from build123d import *

# Parameters (mm, degrees)
F1_DEPTH = 180
F2_R     = 6.5
F3_DEPTH = 25


with BuildPart() as f1:
    # F0 (on Right) → F1 (new body, symmetric)
    with BuildSketch(Plane.YZ):
        Polygon((-50, 0), (0, 0), (0, 50), (-5, 50), (-5, 5), (-45, 5), (-45, 50), (-50, 50), align=None)
    extrude(amount=F1_DEPTH, both=True)

    # F2 (on face) → F3 (cut)
    with BuildSketch(Plane(origin=(0, 0, 0), x_dir=(1, 0, 0), z_dir=(0, 0, -1))):
        with Locations((-60, 25)):
            Circle(F2_R)
        with Locations((60, 25)):
            Circle(F2_R)
    extrude(amount=-F3_DEPTH, mode=Mode.SUBTRACT)


solid = f1.part
Model file for the job. Use its own axes, mm. A direction names the side the tool comes from. Round coordinates to 2 decimals unless told otherwise and drop trailing zeros. Order: outer loops, then holes, each group sorted by start corner. A loop starts at its lowest first (then second) coordinate and runs counter-clockwise, first axis right, second up.
(1) Pin check, flat tip, straight feed: pin 1 (8 mm diameter, centred on x = 113, y = -19, fed in from +Z). Stop position of the tip, or through.
(2) Drill centre lines: line 1 (X direction, y = -25, z = 2.1); line 2 (Y direction, x = 60, z = 2.6); line 3 (Y direction, x = -85, z = 20). Where is each one in solid material? Low to high.
(3) 3-axis set-ups, long thin cutter, end or side, ignore diameter. For faces 1 (the face through (-180, -25.1, 4.7)), 2 (the face through (3, -45, 27)): which of +Z, -Z, +X, -X, +Y, -Y reach the whole face in a straight line?
(4) Band-saw the part on C-C (z = 15). List the corners of the cut face in (x, y).
(5) Pull direction Y, two halves, no side cores. Call faces 3 (the face through (3, -50, 25)), 4 (the face through (3, -25, 0)), 5 (the face through (-53.8, -26.95, 2.46)): released by +Y, released by -Y, zero draft, split by the parting line, or undercut.
(6) Band-saw the part on B-B (x = -60). List the corners of the cut face in (y, z), then the cut area to 3 significant figures.
(7) Band-saw the part on A-A (y = -25). List the corners of the cut face in (x, z).
Verdict:
1. pin 1: stops at z = 5
2. line 1: x = -180 to -66.5, -53.5 to 53.5, 66.5 to 180
2. line 2: y = -50 to -31.5, -18.5 to 0
2. line 3: y = -50 to -45, -5 to 0
3. face 1: +Z, -Z, -X, +Y, -Y
3. face 2: +Z, +X, -X
4. outline: (-180, -50) - (180, -50) - (180, -45) - (-180, -45) - close; (-180, -5) - (180, -5) - (180, 0) - (-180, 0) - close
5. face 3: released by -Y
5. face 4: zero draft
5. face 5: undercut
6. outline: (-50, 0) - (-31.5, 0) - (-31.5, 5) - (-45, 5) - (-45, 50) - (-50, 50) - close; (-18.5, 0) - (0, 0) - (0, 50) - (-5, 50) - (-5, 5) - (-18.5, 5) - close
6. area: 635 mm2
7. outline: (-180, 0) - (-66.5, 0) - (-66.5, 5) - (-180, 5) - close; (-53.5, 0) - (53.5, 0) - (53.5, 5) - (-53.5, 5) - close; (66.5, 0) - (180, 0) - (180, 5) - (66.5, 5) - close
